Input: dimensioned drawing with shaded views. Units: mm. Origin: part minimum x, y, z. A direction names the side the tool comes from. Give positions to 0.01 mm unless a question says otherwise; leave off trailing zeros. Write each loop counter-clockwise with the first axis right and the second up, starting at its lowest first coordinate (ties: lowest second). Pieces come first, ordered by that corner, then holes. Notation, with made-up numbers: (-22, 52) - (4, 52) arc R33 cw to (4, 88) - close; hole circle Ø7 at (-23, 48.5). An arc over 180 degrees is marked (long way). Answer as CSV lines item,"result".
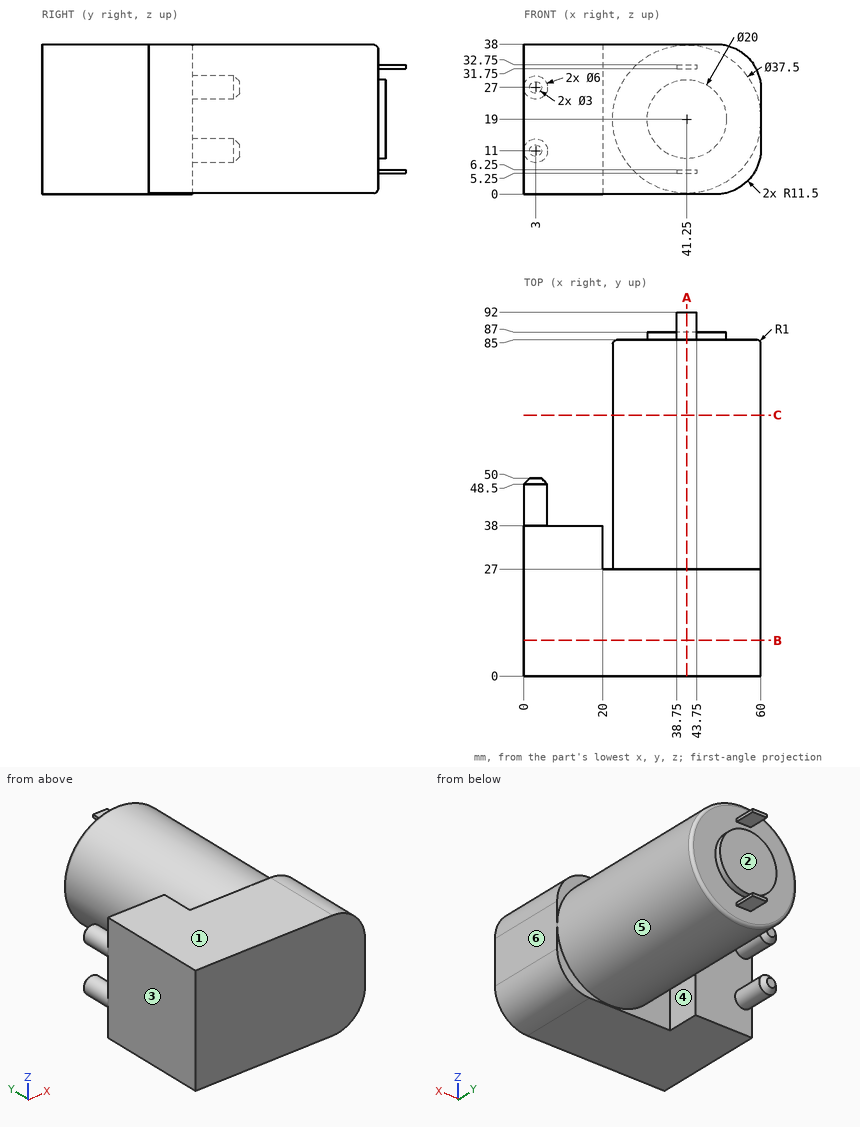
Item 1: Contact query for flat-ended pins moving along their axis: pin 1 (12 mm diameter, centred on x = 47, y = 49.5, fed in from -Z); pin 2 (1.5 mm diameter, centred on y = 79.5, z = 29, fed in from +X); pin 3 (10 mm diameter, centred on x = 45.5, z = 21.5, fed in from +Y). Output: stop coordinate, or through.
The answers:
pin 1,"z = 0.25"
pin 2,"x = 57.56"
pin 3,"y = 87"
Item 2: Cut plane C-C on y = 66. Return the cut outline in (x, z), plus the area to 3 significant figures.
The answers:
outline,"circle Ø37.5 at (41.25, 19)"
area,"1,100 mm²"
Item 3: Cut plane A-A on x = 41.25. Return the cut outline in (y, z), plus the area to 3 significant figures.
The answers:
outline,"(0, 0) - (27, 0) - (27, 0.25) - (84, 0.25) arc R1 ccw to (85, 1.25) - (85, 5.25) - (92, 5.25) - (92, 6.25) - (85, 6.25) - (85, 9) - (87, 9) - (87, 29) - (85, 29) - (85, 31.75) - (92, 31.75) - (92, 32.75) - (85, 32.75) - (85, 36.75) arc R1 ccw to (84, 37.75) - (27, 37.75) - (27, 38) - (0, 38) - close"
area,"3,250 mm²"
Item 4: Cut plane B-B on y = 9. Return the cut outline in (x, z), plus the area to 3 significant figures.
The answers:
outline,"(0, 0) - (48.5, 0) arc R11.5 ccw to (60, 11.5) - (60, 26.5) arc R11.5 ccw to (48.5, 38) - (0, 38) - close"
area,"2,220 mm²"
Item 5: Ray query, line 1 (Y direction, x = 15.5, z = 14); line 2 (Y direction, x = 25.5, z = 24.5); line 3 (X direction, y = 48.5, z = 10.5). Return the intervals inside material, ascending. Write a range as from..to.
The answers:
line 1,"0..38"
line 2,"0..85"
line 3,"0.04..5.96, 24.54..57.96"
Item 6: Mould query, pull axis Z, two halves, no side actions, for the marked faces 1, 2 and 3. Classes: +Z half, -Z half, draft (parallel to the pull), parting line (faces both ways), or undercut.
The answers:
face 1,"+Z half"
face 2,"undercut"
face 3,"draft"
Item 7: Reachability of the marked faces 4, 5 and 6 from +Z, -Z, +X, -X, +Y, -Y: full face, straight path, thin tool, end or side. Return the list, or none.
The answers:
face 4,"+Z, -Z, +Y"
face 5,"+Y"
face 6,"+Z, -Z, +X, +Y, -Y"
